The figure shows three views and two pictorial views of one solid part (mm, origin at its lowest corner). Answer the questions. Round coordinates to 2 decimals unless told otherwise and drop trailing zeros. Order: outer loops, then holes, each group sorted by start corner. A loop starts at its lowest first (then second) coordinate and runs counter-clockwise, first axis right, second up. Notation, with made-up numbers: M 85,6 L 102,6 A15 ccw 102,32 Z; hole C 65,23.25 d6. An arc over 180 degrees is marked long. Return JSON: item names as keys, results as strings.
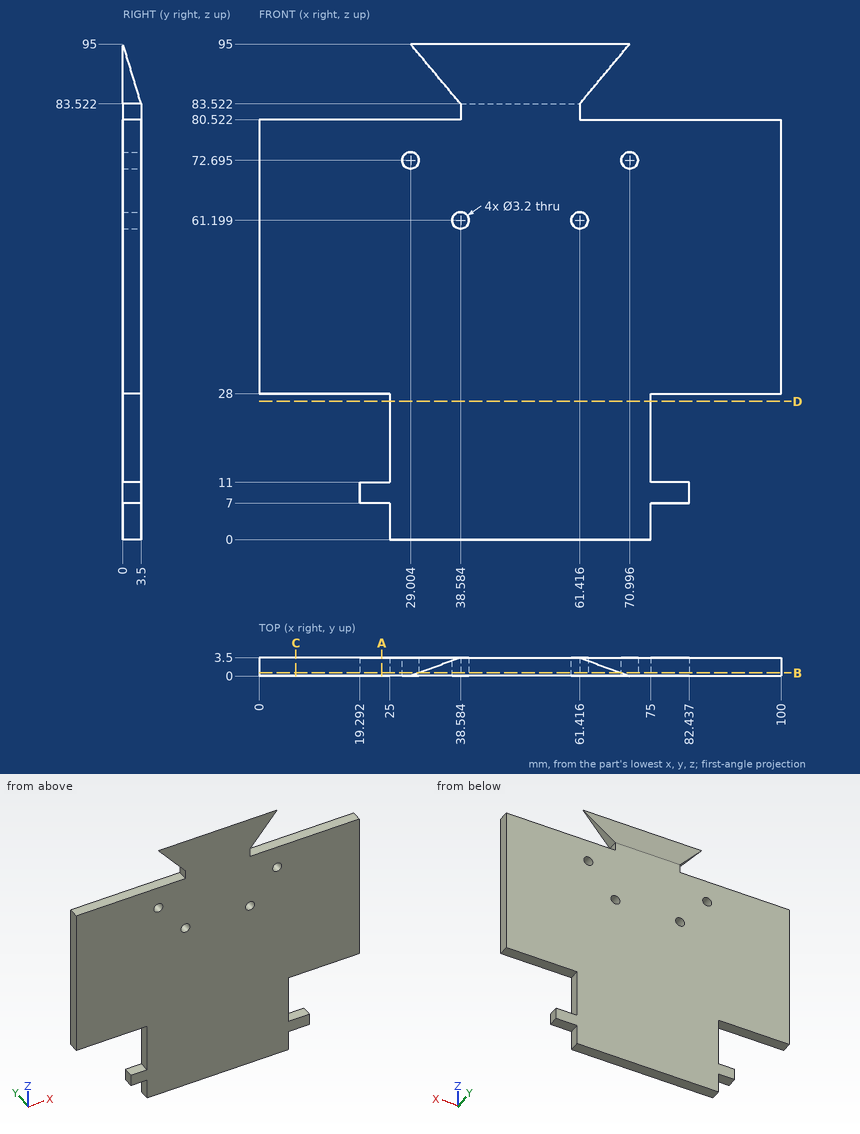
Item 1: Find section A-A (x = 23.5). Determine the outline of the cut face in (y, z), plus the area to 3 significant figures.
Output:
{"outline": "M 0,7 L 3.5,7 L 3.5,11 L 0,11 Z; M 0,28 L 3.5,28 L 3.5,80.52 L 0,80.52 Z", "area": "198 mm^2"}
Item 2: Find section C-C (x = 7). Determine the outline of the cut face in (y, z).
Output:
{"outline": "M 0,28 L 3.5,28 L 3.5,80.52 L 0,80.52 Z"}
Item 3: Consider line 1 along X through (y, z) = (0.2, 72.5); line 2 along Z through (x, y) = (81, 1); line 3 along Z through (x, y) = (29, 3.15) (1 decimal). Determine where each line is inside the solid, lowest interval first. Write a range as [from, to].
Output:
{"line 1": "x = [0, 27.42], [30.59, 69.41], [72.58, 100]", "line 2": "z = [7, 11], [28, 80.52]", "line 3": "z = [0, 71.1], [74.3, 80.5]"}
Item 4: Find section B-B (y = 0.6). Determine the outline of the cut face in (x, z) (1 decimal).
Output:
{"outline": "M 0,28 L 25,28 L 25,11 L 19.3,11 L 19.3,7 L 25,7 L 25,0 L 75,0 L 75,7 L 82.4,7 L 82.4,11 L 75,11 L 75,28 L 100,28 L 100,80.5 L 61.4,80.5 L 61.4,83.5 L 69.4,93 L 30.6,93 L 38.6,83.5 L 38.6,80.5 L 0,80.5 Z; hole C 29,72.7 d3.2; hole C 38.6,61.2 d3.2; hole C 61.4,61.2 d3.2; hole C 71,72.7 d3.2"}
Item 5: Find section D-D (z = 26.5). Determine the outline of the cut face in (x, y).
Output:
{"outline": "M 25,0 L 75,0 L 75,3.5 L 25,3.5 Z"}
Item 6: Each of these flat-tipped pins is pushed along its axis until it touches: pin 1 (1 mm diameter, centred on x = 22.5, y = 2.5, fed in from +Z); pin 2 (1 mm diameter, centred on x = 90, y = 1.5, fed in from -Z); pin 3 (1.8 mm diameter, centred on y = 2.5, z = 9, fed in from -X). Where does it stop, or does it pass through?
Output:
{"pin 1": "stops at z = 80.52", "pin 2": "stops at z = 28", "pin 3": "stops at x = 19.29"}
